The listing builds one solid part. Answer for the finished solid, in the listing's coordinates (mm). A direction names the side the tool comes from. Round coordinates to 2 decimals unless told otherwise and drop trailing zeros. Write each loop counter-clockwise with the first axis right and the second up, starting at its lowest first coordinate (ties: lowest second). Pieces come first, ordered by that corner, then holes. Notation, with made-up numbers: M 30.5,51.5 L 61.5,51.5 A24 cw 61.5,65.5 Z; hole C 41,26.5 d7. An arc over 180 degrees is marked long. One line per item, written item: value. Start each with the question number.
(1) For faces 1 (the flat face through (1, 0, -75)), 2 (the cylindrical face through (56.269, 0.056, 38.396)), determine the directions among +Z, -Z, +X, -X, +Y, -Y from which every point of the face is accessible in a straight line to the end or side of a thin tool.
(2) Section C-C (x = 27.5) is taken. Determine the outline of the cut face in (y, z), plus the area to 3 significant figures.
(3) Consider probe 1 along Z at (x, y) = (31, -1); probe 2 along X at (y, z) = (-0.25, -60.5); probe 3 along Z at (x, y) = (-25, 2.5). Determine where each line is inside the solid, lowest interval first.
(4) For a pull along Z with two mould halves and no side action, classify faces 3 (the flat face through (75, 0, 1)), 4 (the cylindrical face through (69.87, -0.06, 65.59)), 5 (the flat face through (72, 0, -71)) as released by +Z, released by -Z, zero draft, split by the parting line, or undercut.
(5) Section A-A (z = 0) is taken. Determine the outline of the cut face in (x, y).
(6) Section B-B (x = -17) is taken. Determine the outline of the cut face in (y, z).
(7) Section D-D (y = 0.5) is taken. State how many separate pieces and enclosed holes the cut face has, plus the area to 3 significant figures.
```python
from build123d import *

# Parameters (mm, degrees)
SKETCH1_R           = 11.5
SKETCH1_R_2         = 14
SKETCH1_R_3         = 1.5
BOSS_EXTRUDE1_DEPTH = 4


with BuildPart() as part:
    # Sketch1 → Boss-Extrude1 (new, symmetric)
    with BuildSketch(Plane(origin=(0, 0, 0), x_dir=(1, 0, 0), z_dir=(0, 1, 0))):
        Polygon((-68, -75), (68, -75), (75, -68), (75, 68), (68, 75), (-68, 75), (-75, 68), (-75, -68), align=None)
        with Locations(Location((0, 0, 0), (0, 0, 270))):
            Circle(SKETCH1_R, mode=Mode.SUBTRACT)
        with Locations(Location((-58.064971157, 58.064971157, 0), (0, 0, 270))):
            Circle(SKETCH1_R_2, mode=Mode.SUBTRACT)
        with Locations(Location((58.064971157, 58.064971157, 0), (0, 0, 90))):
            Circle(SKETCH1_R_2, mode=Mode.SUBTRACT)
        with Locations(Location((58.064971157, -58.064971157, 0), (0, 0, 270))):
            Circle(SKETCH1_R_2, mode=Mode.SUBTRACT)
        with Locations(Location((-58.064971157, -58.064971157, 0), (0, 0, 90))):
            Circle(SKETCH1_R_2, mode=Mode.SUBTRACT)
        with Locations(Location((-12.85, 7.418950959, 0), (0, 0, 270))):
            Circle(SKETCH1_R_3, mode=Mode.SUBTRACT)
        with Locations(Location((12.85, 7.418950959, 0), (0, 0, 270))):
            Circle(SKETCH1_R_3, mode=Mode.SUBTRACT)
        with Locations(Location((0, -14.837901918, 0), (0, 0, 270))):
            Circle(SKETCH1_R_3, mode=Mode.SUBTRACT)
        with BuildLine():
            Line((-65, -32.380987139), (-65, 32.380987139))
            ThreePointArc((-65, 32.380987139), (-63.793934553, 35.637681876), (-60.757575758, 37.323261815))
            ThreePointArc((-60.757575758, 37.323261815), (-56.330087552, 38.376089353), (-52.1316343, 40.132246498))
            ThreePointArc((-52.1316343, 40.132246498), (-49.06707081, 40.632452823), (-46.298177948, 39.227110136))
            Line((-46.298177948, 39.227110136), (-21.649754839, 14.578687027))
            ThreePointArc((-21.649754839, 14.578687027), (-20.271607616, 11.968214073), (-20.606145336, 9.035307099))
            ThreePointArc((-20.606145336, 9.035307099), (-22.5, 0), (-20.606145336, -9.035307099))
            ThreePointArc((-20.606145336, -9.035307099), (-20.271607616, -11.968214073), (-21.649754839, -14.578687027))
            Line((-21.649754839, -14.578687027), (-46.298177948, -39.227110136))
            ThreePointArc((-46.298177948, -39.227110136), (-49.06707081, -40.632452823), (-52.1316343, -40.132246498))
            ThreePointArc((-52.1316343, -40.132246498), (-56.330087552, -38.376089353), (-60.757575758, -37.323261815))
            ThreePointArc((-60.757575758, -37.323261815), (-63.793934553, -35.637681876), (-65, -32.380987139))
        make_face(mode=Mode.SUBTRACT)
        with BuildLine():
            Line((-32.380987139, 65), (32.380987139, 65))
            ThreePointArc((32.380987139, 65), (35.637681876, 63.793934553), (37.323261815, 60.757575758))
            ThreePointArc((37.323261815, 60.757575758), (38.376089353, 56.330087552), (40.132246498, 52.1316343))
            ThreePointArc((40.132246498, 52.1316343), (40.632452823, 49.06707081), (39.227110136, 46.298177948))
            Line((39.227110136, 46.298177948), (14.578687027, 21.649754839))
            ThreePointArc((14.578687027, 21.649754839), (11.968214073, 20.271607616), (9.035307099, 20.606145336))
            ThreePointArc((9.035307099, 20.606145336), (0, 22.5), (-9.035307099, 20.606145336))
            ThreePointArc((-9.035307099, 20.606145336), (-11.968214073, 20.271607616), (-14.578687027, 21.649754839))
            Line((-14.578687027, 21.649754839), (-39.227110136, 46.298177948))
            ThreePointArc((-39.227110136, 46.298177948), (-40.632452823, 49.06707081), (-40.132246498, 52.1316343))
            ThreePointArc((-40.132246498, 52.1316343), (-38.376089353, 56.330087552), (-37.323261815, 60.757575758))
            ThreePointArc((-37.323261815, 60.757575758), (-35.637681876, 63.793934553), (-32.380987139, 65))
        make_face(mode=Mode.SUBTRACT)
        with BuildLine():
            Line((65, -32.380987139), (65, 32.380987139))
            ThreePointArc((65, 32.380987139), (63.793934553, 35.637681876), (60.757575758, 37.323261815))
            ThreePointArc((60.757575758, 37.323261815), (56.330087552, 38.376089353), (52.1316343, 40.132246498))
            ThreePointArc((52.1316343, 40.132246498), (49.06707081, 40.632452823), (46.298177948, 39.227110136))
            Line((46.298177948, 39.227110136), (21.649754839, 14.578687027))
            ThreePointArc((21.649754839, 14.578687027), (20.271607616, 11.968214073), (20.606145336, 9.035307099))
            ThreePointArc((20.606145336, 9.035307099), (22.5, 0), (20.606145336, -9.035307099))
            ThreePointArc((20.606145336, -9.035307099), (20.271607616, -11.968214073), (21.649754839, -14.578687027))
            Line((21.649754839, -14.578687027), (46.298177948, -39.227110136))
            ThreePointArc((46.298177948, -39.227110136), (49.06707081, -40.632452823), (52.1316343, -40.132246498))
            ThreePointArc((52.1316343, -40.132246498), (56.330087552, -38.376089353), (60.757575758, -37.323261815))
            ThreePointArc((60.757575758, -37.323261815), (63.793934553, -35.637681876), (65, -32.380987139))
        make_face(mode=Mode.SUBTRACT)
        with BuildLine():
            Line((-32.380987139, -65), (32.380987139, -65))
            ThreePointArc((32.380987139, -65), (35.637681876, -63.793934553), (37.323261815, -60.757575758))
            ThreePointArc((37.323261815, -60.757575758), (38.376089353, -56.330087552), (40.132246498, -52.1316343))
            ThreePointArc((40.132246498, -52.1316343), (40.632452823, -49.06707081), (39.227110136, -46.298177948))
            Line((39.227110136, -46.298177948), (14.578687027, -21.649754839))
            ThreePointArc((14.578687027, -21.649754839), (11.968214073, -20.271607616), (9.035307099, -20.606145336))
            ThreePointArc((9.035307099, -20.606145336), (0, -22.5), (-9.035307099, -20.606145336))
            ThreePointArc((-9.035307099, -20.606145336), (-11.968214073, -20.271607616), (-14.578687027, -21.649754839))
            Line((-14.578687027, -21.649754839), (-39.227110136, -46.298177948))
            ThreePointArc((-39.227110136, -46.298177948), (-40.632452823, -49.06707081), (-40.132246498, -52.1316343))
            ThreePointArc((-40.132246498, -52.1316343), (-38.376089353, -56.330087552), (-37.323261815, -60.757575758))
            ThreePointArc((-37.323261815, -60.757575758), (-35.637681876, -63.793934553), (-32.380987139, -65))
        make_face(mode=Mode.SUBTRACT)
    extrude(amount=BOSS_EXTRUDE1_DEPTH, both=True)


solid = part.part
```
Recorded:
1. face 1: -Z, +X, -X, +Y, -Y
1. face 2: +Y, -Y
2. outline: M -4,-75 L 4,-75 L 4,-65 L -4,-65 Z; M -4,-34.57 L 4,-34.57 L 4,-20.43 L -4,-20.43 Z; M -4,20.43 L 4,20.43 L 4,34.57 L -4,34.57 Z; M -4,65 L 4,65 L 4,75 L -4,75 Z
2. area: 386 mm2
3. probe 1: z = -75 to -65, -38.07 to -23.93, 23.93 to 38.07, 65 to 75
3. probe 2: x = -75 to -71.85, -44.28 to -37.36, 37.36 to 44.28, 71.85 to 75
3. probe 3: z = -75 to -65, -32.07 to -17.93, 17.93 to 32.07, 65 to 75
4. face 3: zero draft
4. face 4: undercut
4. face 5: released by -Z
5. outline: M -75,-4 L -65,-4 L -65,4 L -75,4 Z; M -22.5,-4 L -11.5,-4 L -11.5,4 L -22.5,4 Z; M 11.5,-4 L 22.5,-4 L 22.5,4 L 11.5,4 Z; M 65,-4 L 75,-4 L 75,4 L 65,4 Z
6. outline: M -4,-75 L 4,-75 L 4,-65 L -4,-65 Z; M -4,-24.07 L 4,-24.07 L 4,24.07 L -4,24.07 Z; M -4,65 L 4,65 L 4,75 L -4,75 Z
7. separate pieces: 1
7. enclosed holes: 12
7. area: 8,400 mm2
